For this review, use the dimensioned drawing (mm, ordinates from the lowest corner) and the shaded views. A direction names the side the tool comes from. Give positions to 0.01 mm unless a question says otherwise; leave off trailing zeros. Loops run counter-clockwise (first coordinate to the right, second up) from the corner with the lowest first, then second, coordinate; pieces in that order, holes last. Notation, with made-up numbers: (58.25, 76.5) - (84.25, 76.5) arc R20 cw to (84.25, 87.5) - close; hole circle Ø8 at (31, 72.5). An arc over 180 degrees is marked (long way). Put each result on its own line as item: value.
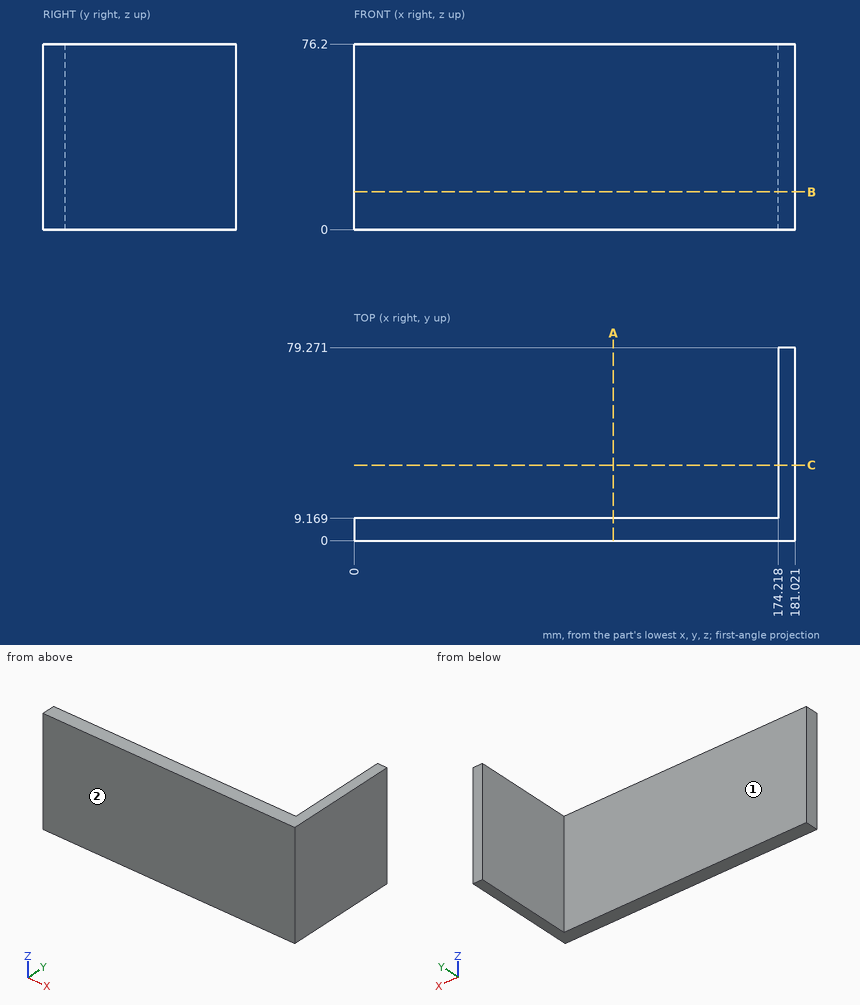
1) Insertion check: pin 1 Ø23 at (x, z) = (110, 20) entering from +Y; pin 2 Ø3 at (y, z) = (64, 11.5) entering from -X. Each pin has a flat end and moves straight along its axis. Give the tip position at first contact, or say it passes through.
Geometry check:
pin 1: stops at y = 9.17
pin 2: stops at x = 174.22
2) For the marked faces 1 and 2, list the 3-axis set-ups (+Z, -Z, +X, -X, +Y, -Y) from which the entire face can be reached by the end or side of a thin tool; tool diameter is ignored.
Geometry check:
face 1: +Z, -Z, -X, +Y
face 2: +Z, -Z, +X, -X, -Y
3) Take a section at C-C on y = 31. State the section outline as (x, z) points.
Geometry check:
outline: (174.22, 0) - (181.02, 0) - (181.02, 76.2) - (174.22, 76.2) - close
4) Take a section at A-A on x = 106.5. State the section outline as (y, z) points, and give its area (3 significant figures).
Geometry check:
outline: (0, 0) - (9.17, 0) - (9.17, 76.2) - (0, 76.2) - close
area: 699 mm²
5) Take a section at B-B on z = 15.5. State the section outline as (x, y) points, and give its area (3 significant figures).
Geometry check:
outline: (0, 0) - (181.02, 0) - (181.02, 79.27) - (174.22, 79.27) - (174.22, 9.17) - (0, 9.17) - close
area: 2,140 mm²
6) Wall thickness on line 1 (X direction, y = 58.5, z = 59.5); line 2 (Y direction, x = 18, z = 3.5): over which ranges is each line inside the solid? List them lowest first.
Geometry check:
line 1: x = 174.22 to 181.02
line 2: y = 0 to 9.17
